```python
from build123d import *

# Parameters (mm, degrees)
SKETCH1_W       = 7.96
SKETCH1_H       = 7.96
EXTRUDE1_DEPTH  = 3.22
SKETCH2_R       = 2.425
EXTRUDE2_DEPTH  = 1.8
LPATTERN1_COUNT = 2
LPATTERN1_PITCH = 7.96
SHELL1_T        = -1.55
SKETCH4_W       = 12.82
SKETCH4_H       = 4.86
EXTRUDE3_DEPTH  = 0.14
SKETCH5_R       = 1.5
SKETCH5_R_2     = 0.64
EXTRUDE4_DEPTH  = 1.81
EXTRUDE5_DEPTH  = 2
EXTRUDE6_DEPTH  = 2
SKETCH8_R       = 1.3
EXTRUDE7_DEPTH  = 15.92


with BuildPart() as part:
    # Sketch1 → Extrude1 (new body)
    with BuildSketch(Plane(origin=(0, 0, 0), x_dir=(1, 0, 0), z_dir=(0, 1, 0))):
        Rectangle(SKETCH1_W, SKETCH1_H)
    extrude1 = extrude(amount=EXTRUDE1_DEPTH)

    # Sketch2 → Extrude2 (add)
    with BuildSketch(Plane(origin=(0, 3.22, 0), x_dir=(1, 0, 0), z_dir=(0, 1, 0))):
        Circle(SKETCH2_R)
    extrude2 = extrude(amount=EXTRUDE2_DEPTH)

    # LPattern1: Extrude1, Extrude2 ×2
    with Locations(*[(i * LPATTERN1_PITCH, 0, 0) for i in range(1, LPATTERN1_COUNT)]):
        add(extrude1)
        add(extrude2)

    # Shell1
    shell1_openings = [part.faces().sort_by_distance(p)[0] for p in [
        (3.98, 0, 0),
    ]]
    offset(amount=SHELL1_T, openings=shell1_openings, kind=Kind.INTERSECTION)

    # Sketch4 → Extrude3 (cut)
    with BuildSketch(Plane.XZ.offset(-1.67)):
        with Locations((3.98, 0)):
            Rectangle(SKETCH4_W, SKETCH4_H)
    extrude(amount=-EXTRUDE3_DEPTH, mode=Mode.SUBTRACT)

    # Sketch5 → Extrude4 (add)
    with BuildSketch(Plane.XZ.offset(-1.81)):
        with Locations((3.98, 0)):
            Circle(SKETCH5_R)
        with Locations((3.98, 0)):
            Circle(SKETCH5_R_2, mode=Mode.SUBTRACT)
    extrude(amount=EXTRUDE4_DEPTH)

    # Sketch6 → Extrude5 (add)
    with BuildSketch(Plane(origin=(11.94, 0, 0), x_dir=(0, 0, -1), z_dir=(1, 0, 0))):
        with BuildLine():
            Line((-7.73, 0), (-3.98, 0))
            Line((-3.98, 0), (-3.98, 3.22))
            Line((-3.98, 3.22), (-5.699827594, 3.22))
            ThreePointArc((-5.699827594, 3.22), (-9.633286631, 3.45), (-7.73, 0))
        make_face()
    extrude(amount=-EXTRUDE5_DEPTH)

    # Sketch7 → Extrude6 (add)
    with BuildSketch(Plane.ZY.offset(3.98)):
        with BuildLine():
            Line((3.98, 3.22), (3.98, 0))
            Line((3.98, 0), (7.73, 0))
            ThreePointArc((7.73, 0), (9.633286631, 3.45), (5.699827594, 3.22))
            Line((5.699827594, 3.22), (3.98, 3.22))
        make_face()
    extrude(amount=-EXTRUDE6_DEPTH)

    # Sketch8 → Extrude7 (add)
    with BuildSketch(Plane.ZY.offset(3.98)):
        with Locations((7.73, 2.25)):
            Circle(SKETCH8_R)
    extrude(amount=-EXTRUDE7_DEPTH)


solid = part.part
```
Here's how the part is built. I have some questions about the finished solid (model axes, mm). A direction names the side the tool comes from. Give positions to 0.01 mm unless a question says otherwise; leave off trailing zeros. Loops run counter-clockwise (first coordinate to the right, second up) from the corner with the lowest first, then second, coordinate; pieces in that order, holes last. Notation, with made-up numbers: M -22,86.5 L 9,86.5 A17 cw 9,90.5 Z; hole C -20.5,-8 d6. An arc over 180 degrees is marked long. Return JSON: item names as keys, results as strings.
Item 1: Thinking about a two-plate mould opening in Z: for faces 5 (the flat face through (0, 5.02, 0)), 6 (the flat face through (0, 3.47, 0)), which applies, released by +Z, released by -Z, zero draft, split by the parting line, or undercut?
A:
{"face 5": "zero draft", "face 6": "undercut"}
Item 2: Imagine slicing it at D-D on x = 0. List the corners of the cut face in (y, z) for me (3 decimals), then the cut area to 3 significant figures.
A:
{"outline": "M 0,-3.98 L 3.22,-3.98 L 3.22,-2.425 L 5.02,-2.425 L 5.02,2.425 L 3.22,2.425 L 3.22,3.98 L 0,3.98 L 0,2.43 L 1.81,2.43 L 1.81,0.875 L 3.47,0.875 L 3.47,-0.875 L 1.81,-0.875 L 1.81,-2.43 L 0,-2.43 Z; C 2.25,7.73 d2.6", "area": "28.0 mm^2"}
Item 3: Imagine slicing it at C-C on y = 2.25. List the corners of the cut face in (x, z) for me (3 decimals).
A:
{"outline": "M -3.98,-3.98 L 11.94,-3.98 L 11.94,9.98 L 9.94,9.98 L 9.94,9.03 L -1.98,9.03 L -1.98,9.98 L -3.98,9.98 Z; hole M -1.98,3.98 L 9.94,3.98 L 9.94,6.43 L -1.98,6.43 Z; hole C 0,0 d1.75; hole C 7.96,0 d1.75"}
Item 4: Please list where these lines run through material, in increasing order: line 1 (Z direction, x = 4.5, y = 0.5); line 2 (X direction, y = 0.9, z = 1); line 3 (X direction, y = 3.2, z = 6.5).
A:
{"line 1": "z = -3.98 to -2.43, -1.41 to -0.37, 0.37 to 1.41, 2.43 to 3.98", "line 2": "x = -3.98 to -2.43, 2.86 to 5.1, 10.39 to 11.94", "line 3": "x = -3.98 to -1.98, 9.94 to 11.94"}
Item 5: Imagine slicing it at A-A on x = 3.98. List the corners of the cut face in (y, z) for me, then the cut area to 3 significant figures.
A:
{"outline": "M 0,-3.98 L 3.22,-3.98 L 3.22,3.98 L 0,3.98 L 0,2.43 L 1.81,2.43 L 1.81,1.5 L 0,1.5 L 0,0.64 L 1.81,0.64 L 1.81,-0.64 L 0,-0.64 L 0,-1.5 L 1.81,-1.5 L 1.81,-2.43 L 0,-2.43 Z; C 2.25,7.73 d2.6", "area": "25.3 mm^2"}
Item 6: I'm going to push flat-ended pins straight in: pin 1 Ø1.9 at (x, z) = (8.5, -0.5) entering from -Y; pin 2 Ø1.6 at (x, y) = (2, 2) entering from +Z; pin 3 Ø0.5 at (x, y) = (1.5, 1) entering from +Z. Where does each tip first touch, or does it pass through?
A:
{"pin 1": "stops at y = 1.81", "pin 2": "stops at z = 9.03", "pin 3": "stops at z = 8.56"}
Item 7: On a 3-axis mill with a long thin cutter (end or side, diameter ignored), from which of +Z, -Z, +X, -X, +Y, -Y can I reach the whole of each face in a straight line? I mean faces 1 (the flat face through (4, 2, 3.98)), 2 (the cylindrical face through (2.313, 4.107, -0.728)), 3 (the flat face through (9.94, 2, 6)), 4 (the flat face through (10.39, 1, 0)). Say none if no direction works.
A:
{"face 1": "+Y, -Y", "face 2": "+Y", "face 3": "none", "face 4": "-Y"}
